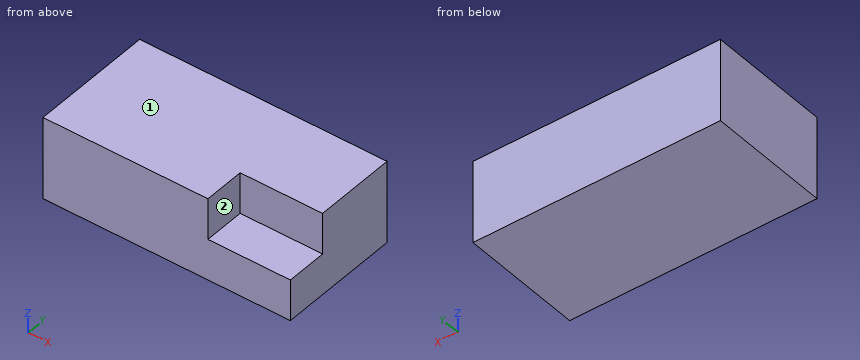
from build123d import *

# Parameters (mm, degrees)
F0_W     = 25.4
F0_H     = 25.4
F1_DEPTH = 152.4
F3_W     = 50.8
F3_H     = 25.4
F4_DEPTH = 25.4


with BuildPart() as f1:
    # F0 (on Right) → F1 (new body)
    with BuildSketch(Plane.YZ):
        Polygon((0, 25.4), (0, 0), (76.2, 0), (76.2, 50.8), (25.4, 50.8), (25.4, 25.4), align=None)
        with Locations((12.7, 38.1)):
            Rectangle(F0_W, F0_H)
    extrude(amount=F1_DEPTH)

    # F3 (on face) → F4 (cut)
    with BuildSketch(Plane.XY.offset(50.8)):
        with Locations((127, 12.7)):
            Rectangle(F3_W, F3_H)
    extrude(amount=-F4_DEPTH, mode=Mode.SUBTRACT)


solid = f1.part
Source: CAD feature listing. Evaluate the final solid. Frame: model axes, mm. Face numbers are marked on the shaded views. A direction names the side the tool comes from. Round coordinates to 2 decimals unless told otherwise and drop trailing zeros. Loops run counter-clockwise (first coordinate to the right, second up) from the corner with the lowest first, then second, coordinate; pieces in that order, holes last. Notation, with made-up numbers: (43, 62.25) - (51, 62.25) arc R9 cw to (51, 79.25) - close; hole circle Ø1 at (41, -12). An arc over 180 degrees is marked (long way). Write item = value, one per line. Start each with the question number.
(1) Section query B-B, the plane z = 47. Output: boundary loops of the cut face in (x, y).
(2) Pin query (flat end, axial travel): pin 1 (12.5 mm diameter, centred on x = 114.5, z = 41, fed in from -Y); pin 2 (7.5 mm diameter, centred on y = 8.5, z = 42.5, fed in from +X). Return the tip coordinate at first contact, or that it passes through.
(3) Ray query, line 1 along Y through (x, z) = (133, 32.5); line 2 along X through (y, z) = (23.5, 49). Return the intervals inside material, ascending. Write a range as from..to.
(4) Set-up query: the marked faces 1 and 2. Return all of +Z, -Z, +X, -X, +Y, -Y with unobstructed straight access to the full face (end or side cutting, diameter ignored); none if empty.
(5) Section query A-A, the plane y = 19. Output: boundary loops of the cut face in (x, z).
Conclusion:
q1.outline = (0, 0) - (101.6, 0) - (101.6, 25.4) - (152.4, 25.4) - (152.4, 76.2) - (0, 76.2) - close
q2.pin_1 = 25.4
q2.pin_2 = 101.6
q3.line_1 = 25.4..76.2
q3.line_2 = 0..101.6
q4.face_1 = +Z, +X, -X, +Y, -Y
q4.face_2 = +Z, +X, -Y
q5.outline = (0, 0) - (152.4, 0) - (152.4, 25.4) - (101.6, 25.4) - (101.6, 50.8) - (0, 50.8) - close
